Autodesk Inventor part; units mm, degrees
ref_plane "YZ Plane" through (0, 0, 0) normal (1, 0, 0) x (0, 1, 0)
ref_plane "XZ Plane" through (0, 0, 0) normal (0, 1, 0) x (-1, 0, 0)
ref_plane "XY Plane" through (0, 0, 0) normal (0, 0, 1) x (1, 0, 0)
sketch "Sketch1" plane through (0, 0, 0) normal (1, 0, 0) x (0, 1, 0)
  line L0 (0, 0) -> (850, 0)
  line L1 (850, 0) -> (850, -175)
  line L2 (850, -175) -> (0, -175)
  line L3 (0, -175) -> (0, 0)
  dimension "d0" = 850
  dimension "d1" = 175
extrude "Extrusion1" add sketch "Sketch1" along normal blind 50
sketch "Sketch2" plane through (50, 0, 0) normal (1, 0, 0) x (0, 0, -1)
  line L0 (0, 0) -> (175, 0)
  line L1 (175, 850) -> (0, 850)
  line L2 (10, 0) -> (165, 0)
  line L3 (165, 0) -> (165, 850)
  line L4 (165, 850) -> (10, 850)
  line L5 (10, 850) -> (10, 0)
  dimension "d4" = 155
extrude "Extrusion2" cut sketch "Sketch2" against normal blind 40
fillet "Fillet1" radius 4 2 edges at (10, 425, -165) (10, 425, -10)
equation "\"BendRadius\" = Thickness"
equation "\"BendReliefWidth\" = Thickness"
equation "\"BendReliefDepth\" = 0.5 * Thickness"
equation "\"CornerReliefSize\" = 4 * Thickness"
equation "\"MinimumRemnant\" = 2 * Thickness"
equation "\"TransitionRadius\" = BendRadius"
equation "\"JacobiRadiusSize\" = BendRadius"
equation "\"GapSize\" = Thickness"
properties part number "Base2"
Source: CAD feature listing. Evaluate the final solid. Frame: model axes, mm. A direction names the side the tool comes from. Coordinates: 2 decimals unless noted, no trailing zeros. Loops run counter-clockwise (first coordinate to the right, second up) from the corner with the lowest first, then second, coordinate; pieces in that order, holes last. Notation, with made-up numbers: M -11.5,83 L 15.5,83 A21 cw 15.5,97 Z; hole C 41.25,50 d8. An arc over 180 degrees is marked long. Use CSV: the item, a comma, the result in double quotes.
(1) Draft query along Z for faces 1 (the face through (32, 431, -10)), 2 (the face through (8, 850, -81)), 3 (the face through (25, 431, -175)). Return one class per face: pulls with the +Z half, pulls with the -Z half, needs draft (parallel to the pull), parting line crosses it, or undercut.
Answers follow:
face 1,"undercut"
face 2,"needs draft"
face 3,"pulls with the -Z half"
(2) Line query: line 1 (Z direction, x = 40, y = 744.5); line 2 (X direction, y = 545, z = -60); line 3 (Z direction, x = 11.5, y = 236.5). Output: solid intervals per line, ascending. Write a range as [from, to].
Answers follow:
line 1,"[-175, -165], [-10, 0]"
line 2,"[0, 10]"
line 3,"[-175, -164.12], [-10.88, 0]"
(3) Cut plane C-C on z = -126. Return loops of the section in (x, y).
Answers follow:
outline,"M 0,0 L 10,0 L 10,850 L 0,850 Z"
(4) Contact query for flat-ended pins moving along their axis: pin 1 (6 mm diameter, centred on x = 14.5, z = -67, fed in from -Y); pin 2 (10 mm diameter, centred on y = 328.5, z = -91.5, fed in from +X). Output: stop coordinate, or through.
Answers follow:
pin 1,"through"
pin 2,"x = 10"
(5) Cut plane A-A on x = 26.5. Return loops of the section in (y, z), and give its area (3 significant figures).
Answers follow:
outline,"M 0,-175 L 850,-175 L 850,-165 L 0,-165 Z; M 0,-10 L 850,-10 L 850,0 L 0,0 Z"
area,"17,000 mm²"
(6) Cut plane B-B on y = 454.5. Return loops of the section in (x, z), and give its area (3 significant figures).
Answers follow:
outline,"M 0,-175 L 50,-175 L 50,-165 L 14,-165 A4 cw 10,-161 L 10,-14 A4 cw 14,-10 L 50,-10 L 50,0 L 0,0 Z"
area,"2,560 mm²"
(7) Reachability of faces 4 (the face through (25, 419, 0)), 5 (the face through (10, 431, -86)) from +Z, -Z, +X, -X, +Y, -Y: full face, straight path, thin tool, end or side. Return the list, or none.
Answers follow:
face 4,"+Z, +X, -X, +Y, -Y"
face 5,"+X, +Y, -Y"
